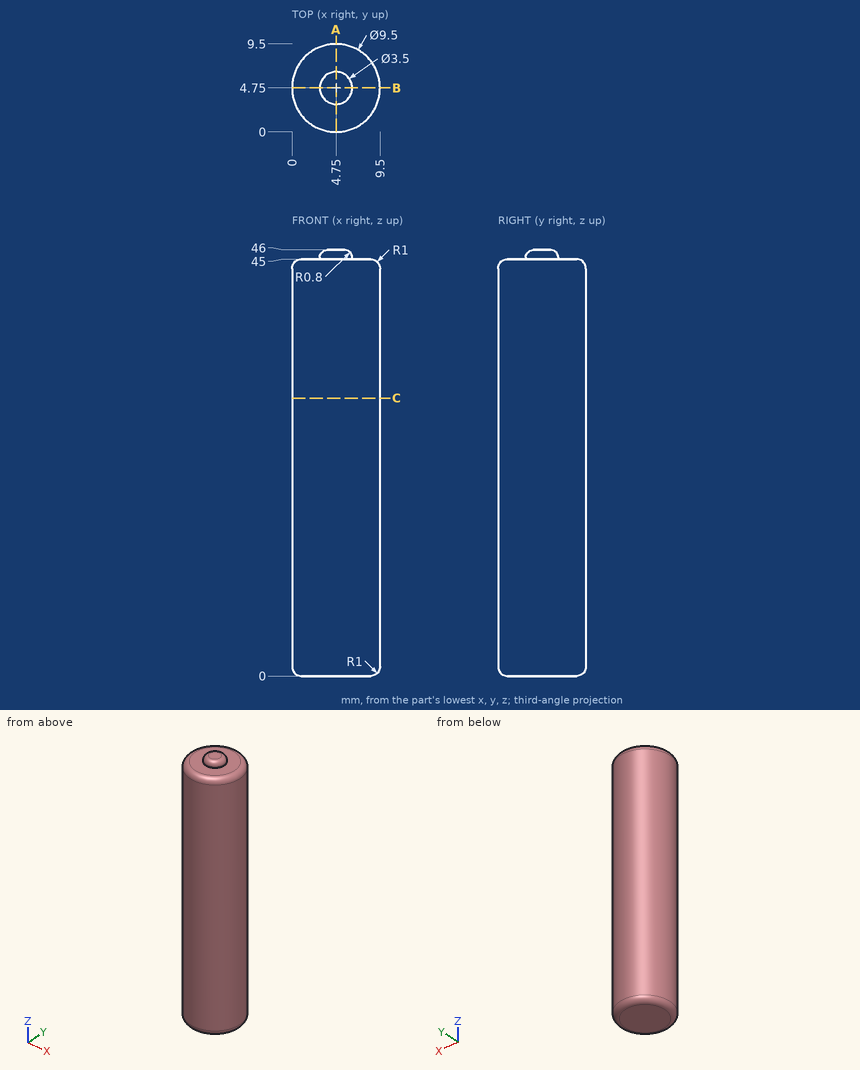
The drawing under review shows one solid part. Ordinate dimensions are in mm from its lowest x, y, z. Give positions to 0.01 mm unless a question says otherwise; leave off trailing zeros. Write each loop counter-clockwise with the first axis right and the second up, starting at its lowest first coordinate (ties: lowest second). Pieces come first, ordered by that corner, then holes.
1. Wall thickness on L1, parallel to Z at x = 8, y = 6.5; L2, parallel to X at y = 4.5, z = 22; L3, parallel to Y at x = 7.5, z = 3: over which ranges is each line inside the solid? List them lowest first.
2. Add section A-A, the plane x = 4.75. Write out the cut boundary in (y, z).
3. Add section C-C, the plane z = 30. Write out the cut boundary in (x, y).
4. For P1, Ø3, axis at y = 6.5, z = 19, coming from the -X side; P2, Ø1, axis at y = 8, z = 23, coming from the -X side; P3, Ø3, axis at x = 2.5, z = 7, coming from the +Y side; P4, Ø3, axis at y = 6, z = 41, coming from the +X side, all flat-tipped, find the tip position at first contact; note any pin that passes through.
Worked answers:
1. L1: z = 0 to 45
1. L2: x = 0.01 to 9.49
1. L3: y = 0.88 to 8.62
2. outline: (0, 1) arc R1 ccw to (1, 0) - (8.5, 0) arc R1 ccw to (9.5, 1) - (9.5, 44) arc R1 ccw to (8.5, 45) - (6.5, 45) - (6.5, 45.2) arc R0.8 ccw to (5.7, 46) - (3.8, 46) arc R0.8 ccw to (3, 45.2) - (3, 45) - (1, 45) arc R1 ccw to (0, 44) - close
3. outline: circle Ø9.5 at (4.75, 4.75)
4. P1: stops at x = 0.01
4. P2: stops at x = 0.88
4. P3: stops at y = 9.44
4. P4: stops at x = 9.5
